from build123d import *

# Parameters (mm, degrees)
SKETCH_1_W           = 13
SKETCH_1_H           = 5.5
EXTRUDE_1_DEPTH      = 14.5
SKETCH_2_W           = 12.6
SKETCH_2_H           = 5.1
CUT_EXTRUDE_1_DEPTH  = 9
CUT_EXTRUDE_3_DEPTH  = 17.815171721
CUT_EXTRUDE_4_DEPTH  = 20.667549415
SKETCH_5_W           = 10.6
SKETCH_5_H           = 1.1
EXTRUDE_3_DEPTH      = 9
CHAMFER_1_SIZE       = 1
CHAMFER_1_SIZE2      = 0.267949192
SKETCH_3_W           = 13
SKETCH_3_H           = 4
CUT_EXTRUDE_2_DEPTH  = 1.8
SKETCH_9_W           = 0.64
SKETCH_9_H           = 0.25
EXTRUDE_5_DEPTH      = 3.4
SKETCH_14_W          = 0.64
SKETCH_14_H          = 8.130016943
EXTRUDE_6_DEPTH      = 0.1
SKETCH_15_W          = 0.2
SKETCH_15_H          = 1.9
SKETCH_17_W          = 12.6
SKETCH_17_H          = 0.8
SKETCH_17_W_2        = 0.8
SKETCH_17_H_2        = 5.1
EXTRUDE_14_7_1_DEPTH = 0.2


with BuildPart() as part:
    # 草图1 → 凸台-拉伸1 (new body)
    with BuildSketch(Plane.XY):
        Rectangle(SKETCH_1_W, SKETCH_1_H)
    extrude(amount=EXTRUDE_1_DEPTH)

    # 草图2 → 切除-拉伸1 (cut)
    with BuildSketch(Plane.XY.offset(14.5)):
        Rectangle(SKETCH_2_W, SKETCH_2_H)
    extrude(amount=-CUT_EXTRUDE_1_DEPTH, mode=Mode.SUBTRACT)

    # 草图11 → 切除-拉伸3 (cut, through all)
    with BuildSketch(Plane.XZ.offset(2.75)):
        with BuildLine():
            Line((4.75, 7.5), (4.75, 13))
            ThreePointArc((4.75, 13), (4.603553391, 13.353553391), (4.25, 13.5))
            Line((4.25, 13.5), (2.25, 13.5))
            ThreePointArc((2.25, 13.5), (1.896446609, 13.353553391), (1.75, 13))
            Line((1.75, 13), (1.75, 7.5))
            Line((1.75, 7.5), (2.1, 7.5))
            Line((2.1, 7.5), (2.65, 12.5))
            ThreePointArc((2.65, 12.5), (3.25, 13.037619085), (3.85, 12.5))
            Line((3.85, 12.5), (4.4, 7.5))
            Line((4.4, 7.5), (4.75, 7.5))
        make_face()
        with BuildLine():
            Line((-3.85, 12.5), (-4.4, 7.5))
            Line((-4.4, 7.5), (-4.75, 7.5))
            Line((-4.75, 7.5), (-4.75, 13))
            ThreePointArc((-4.75, 13), (-4.603553391, 13.353553391), (-4.25, 13.5))
            Line((-4.25, 13.5), (-2.25, 13.5))
            ThreePointArc((-2.25, 13.5), (-1.896446609, 13.353553391), (-1.75, 13))
            Line((-1.75, 13), (-1.75, 7.5))
            Line((-1.75, 7.5), (-2.1, 7.5))
            Line((-2.1, 7.5), (-2.65, 12.5))
            ThreePointArc((-2.65, 12.5), (-3.25, 13.037619085), (-3.85, 12.5))
        make_face()
    extrude(amount=-CUT_EXTRUDE_3_DEPTH, mode=Mode.SUBTRACT)

    # 草图12 → 切除-拉伸4 (cut, through all)
    with BuildSketch(Plane(origin=(6.5, 0, 0), x_dir=(0, 0, -1), z_dir=(1, 0, 0))):
        with BuildLine():
            Line((-13.5, -1.5), (-7.5, -1.5))
            Line((-7.5, -1.5), (-7.5, 1.5))
            Line((-7.5, 1.5), (-13.5, 1.5))
            Line((-13.5, 1.5), (-13.5, 1.15))
            Line((-13.5, 1.15), (-8.5, 0.6))
            ThreePointArc((-8.5, 0.6), (-7.962380915, 0), (-8.5, -0.6))
            Line((-8.5, -0.6), (-13.5, -1.15))
            Line((-13.5, -1.15), (-13.5, -1.5))
        make_face()
    extrude(amount=-CUT_EXTRUDE_4_DEPTH, mode=Mode.SUBTRACT)

    # 草图5 → 凸台-拉伸3 (add)
    with BuildSketch(Plane.XY.offset(5.5)):
        with Locations((0, -1)):
            Rectangle(SKETCH_5_W, SKETCH_5_H)
    extrude(amount=EXTRUDE_3_DEPTH)

    # 倒角1
    chamfer_1_edges = [part.edges().sort_by_distance(p)[0] for p in [
        (0, -0.45, 14.5),
    ]]
    chamfer_1_side = [part.faces().sort_by_distance(p)[0] for p in [
        (0, -0.45, 10),
    ]]
    chamfer(chamfer_1_edges, length=CHAMFER_1_SIZE, length2=CHAMFER_1_SIZE2, reference=chamfer_1_side[0])

    # 草图3 → 切除-拉伸2 (cut)
    with BuildSketch(Plane(origin=(0, 2.75, 0), x_dir=(1, 0, 0), z_dir=(0, 1, 0))):
        with Locations((0, -2)):
            Rectangle(SKETCH_3_W, SKETCH_3_H)
    extrude(amount=-CUT_EXTRUDE_2_DEPTH, mode=Mode.SUBTRACT)

    # 草图9 → 凸台-拉伸5 (add)
    with BuildSketch(Plane(origin=(0, 0.95, 2.45), x_dir=(-1, 0, 0), z_dir=(0, -1, 0))):
        with Locations((-3.5, 1.525)):
            Rectangle(SKETCH_9_W, SKETCH_9_H)
        with Locations((1, 1.525)):
            Rectangle(SKETCH_9_W, SKETCH_9_H)
        with Locations((-1, 1.525)):
            Rectangle(SKETCH_9_W, SKETCH_9_H)
        with Locations((3.5, 1.525)):
            Rectangle(SKETCH_9_W, SKETCH_9_H)
    extrude(amount=-EXTRUDE_5_DEPTH)

    # 草图14 → 凸台-拉伸6 (add)
    with BuildSketch(Plane(origin=(0, -0.45, 0), x_dir=(1, 0, 0), z_dir=(0, 1, 0))):
        with Locations((-3.5, -9.434991528)):
            Rectangle(SKETCH_14_W, SKETCH_14_H)
        with Locations((-1, -9.434991528)):
            Rectangle(SKETCH_14_W, SKETCH_14_H)
        with Locations((1, -9.434991528)):
            Rectangle(SKETCH_14_W, SKETCH_14_H)
        with Locations((3.5, -9.434991528)):
            Rectangle(SKETCH_14_W, SKETCH_14_H)
    extrude(amount=EXTRUDE_6_DEPTH)

    # 扫描1: sweep along a path in 草图16
    with BuildLine(Plane(origin=(0, 0, 0), x_dir=(-1, 0, 0), z_dir=(0, 0, -1))) as sweep_1_path:
        Line((6.5, 0.95), (7.189615975, 2.293290664))
        ThreePointArc((7.189615975, 2.293290664), (7.3, 2.75), (7.189615975, 3.206709336))
        Line((7.189615975, 3.206709336), (6.602675615, 4.35))
    # 草图15 → 扫描1 (sweep)
    with BuildSketch(Plane(origin=(0, 0.95, 0), x_dir=(1, 0, 0), z_dir=(0, 1, 0))):
        with Locations((-6.4, -2.375)):
            Rectangle(SKETCH_15_W, SKETCH_15_H)
    sweep_1 = sweep(path=sweep_1_path.line)

    # 镜向1: 扫描1 across plane
    add(sweep_1.mirror(Plane(origin=(0, 0, 0), x_dir=(0, 0, 1), z_dir=(1, 0, 0))))

    # 草图17 → 卷边-外径14*7.1 (add)
    with BuildSketch(Plane.XY.offset(14.5)):
        with Locations((0, -3.15)):
            Rectangle(SKETCH_17_W, SKETCH_17_H)
        with Locations((6.9, 0)):
            Rectangle(SKETCH_17_W_2, SKETCH_17_H_2)
        with Locations((-6.9, 0)):
            Rectangle(SKETCH_17_W_2, SKETCH_17_H_2)
        with Locations((0, 3.15)):
            Rectangle(SKETCH_17_W, SKETCH_17_H)
    extrude(amount=-EXTRUDE_14_7_1_DEPTH)


solid = part.part
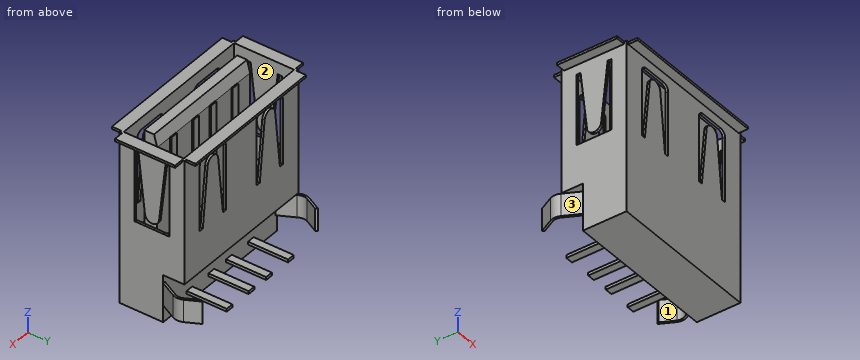
Geometry check sheet. Reference: the model listing, model coordinates, mm. Face numbers are marked on the shaded views. A direction names the side the tool comes from. Give positions to 0.01 mm unless a question says otherwise; leave off trailing zeros. Write each loop counter-clockwise with the first axis right and the second up, starting at its lowest first coordinate (ties: lowest second). Pieces come first, ordered by that corner, then holes. Notation, with made-up numbers: M 47.25,44.5 L 97.25,44.5 A10 ccw 97.25,56.5 Z; hole C -23,35.25 d2. An arc over 180 degrees is marked long. Answer as CSV lines item,"result". Start each with the question number.
Q1. Material ranges on L1, parallel to Y at x = 0.75, z = 10.75; L2, parallel to X at y = -0.5, z = 11.5; L3, parallel to X at y = 0.5, z = 11.5, recorded low to high.
Q2. Section check C-C, the plane z = 11.25. Give the number of separate pieces and of enclosed holes in the cut face, then the cut area to 3 significant figures.
Q3. Go/stop test with flat-tipped pins: pin 1 (0.5 mm diameter, centred on x = 1, z = 8.5, fed in from +Y); pin 2 (1 mm diameter, centred on x = 0, y = 2, fed in from +Z); pin 3 (1 mm diameter, centred on y = 2.5, z = 8, fed in from +X). Record where each tip stops, or that it passes through.
Q4. Section check D-D, the plane y = -3. Record the cut outline in (x, z), then the cut area to 3 significant figures.
Q5. Section check B-B, the plane z = 2. Record the cut outline in (x, y), then the cut area to 3 significant figures.
Q6. Section check A-A, the plane x = 0.5. Record the cut outline in (y, z), then the cut area to 3 significant figures.
Q7. Tool access check on the marked faces 1, 2 and 3. Record the directions out of +Z, -Z, +X, -X, +Y, -Y that give a thin tool (end or side, any length) a straight path to the whole face; none if there is none.
Geometry says:
1,L1,"-2.75 to -2.55, -1.55 to -0.35, 2.55 to 2.75"
1,L2,"-6.5 to -6.3, -5.3 to 5.3, 6.3 to 6.5"
1,L3,"-6.5 to -6.3, 6.3 to 6.5"
2,separate pieces,"13"
2,enclosed holes,"0"
2,area,"17.5 mm^2"
3,pin 1,"y = 2.75"
3,pin 2,"z = 5.5"
3,pin 3,"x = 6.5"
4,outline,"M -6.3,14.3 L 6.3,14.3 L 6.3,14.5 L -6.3,14.5 Z"
4,area,"2.52 mm^2"
5,outline,"M -7.19,2.29 L -6.5,0.95 L -6.5,-2.75 L 6.5,-2.75 L 6.5,0.95 L 7.19,2.29 A1 ccw 7.19,3.21 L 6.6,4.35 L 6.49,4.19 L 7.07,3.04 A0.83 cw 6.99,2.29 L 6.3,0.95 L -6.3,0.95 L -6.99,2.29 A0.83 cw -7.07,3.04 L -6.49,4.19 L -6.6,4.35 L -7.19,3.21 A1 ccw Z"
5,area,"49.4 mm^2"
6,outline,"M -3.55,14.3 L -2.75,14.3 L -2.75,0 L 0.95,0 L 0.95,4 L 2.75,4 L 2.75,14.3 L 3.55,14.3 L 3.55,14.5 L 2.55,14.5 L 2.55,5.5 L -0.45,5.5 L -0.45,13.5 L -0.72,14.5 L -1.55,14.5 L -1.55,5.5 L -2.55,5.5 L -2.55,14.5 L -3.55,14.5 Z"
6,area,"36.7 mm^2"
7,face 1,"+Z, -Z"
7,face 2,"+Z"
7,face 3,"-Z, -X, -Y"
